```python
from build123d import *

# Parameters (mm, degrees)
SKETCH1_W           = 65
SKETCH1_H           = 57
SKETCH1_R           = 3.25
BOSS_EXTRUDE1_DEPTH = 21.5
CHAMFER1_SIZE       = 6
SKETCH2_W           = 13
SKETCH2_H           = 26
SKETCH2_H_2         = 5
CUT_EXTRUDE1_DEPTH  = 19.5
FILLET1_R           = 3


with BuildPart() as part:
    # Sketch1 → Boss-Extrude1 (new body)
    with BuildSketch(Plane(origin=(0, 0, 0), x_dir=(1, 0, 0), z_dir=(0, 1, 0))):
        Rectangle(SKETCH1_W, SKETCH1_H)
        with Locations((27.75, -2.25)):
            Circle(SKETCH1_R, mode=Mode.SUBTRACT)
        with Locations((-27.75, -2.25)):
            Circle(SKETCH1_R, mode=Mode.SUBTRACT)
    extrude(amount=BOSS_EXTRUDE1_DEPTH)

    # Chamfer1
    chamfer1_edges = [part.edges().sort_by_distance(p)[0] for p in [
        (32.5, 10.75, 28.5),
        (-32.5, 10.75, 28.5),
        (-32.5, 10.75, -28.5),
        (32.5, 10.75, -28.5),
    ]]
    chamfer(chamfer1_edges, length=CHAMFER1_SIZE)

    # Sketch2 → Cut-Extrude1 (cut)
    with BuildSketch(Plane(origin=(0, 21.5, 0), x_dir=(1, 0, 0), z_dir=(0, 1, 0))):
        with Locations((-26, 0)):
            Rectangle(SKETCH2_W, SKETCH2_H)
        with Locations((-26, 17.1)):
            Rectangle(SKETCH2_W, SKETCH2_H_2)
        with Locations((-26, 23.7)):
            Rectangle(SKETCH2_W, SKETCH2_H_2)
        with Locations((-26, -17.1)):
            Rectangle(SKETCH2_W, SKETCH2_H_2)
        with Locations((-26, -23.7)):
            Rectangle(SKETCH2_W, SKETCH2_H_2)
        with Locations((26, -23.7)):
            Rectangle(SKETCH2_W, SKETCH2_H_2)
        with Locations((26, -17.1)):
            Rectangle(SKETCH2_W, SKETCH2_H_2)
        with Locations((26, 0)):
            Rectangle(SKETCH2_W, SKETCH2_H)
        with Locations((26, 17.1)):
            Rectangle(SKETCH2_W, SKETCH2_H_2)
        with Locations((26, 23.7)):
            Rectangle(SKETCH2_W, SKETCH2_H_2)
    extrude(amount=-CUT_EXTRUDE1_DEPTH, mode=Mode.SUBTRACT)

    # Fillet1
    fillet1_edges = [part.edges().sort_by_distance(p)[0] for p in [
        (-19.5, 21.5, 17.1),
        (-19.5, 21.5, 23.7),
        (19.5, 21.5, 23.7),
        (19.5, 21.5, 17.1),
        (19.5, 21.5, 0),
        (19.5, 21.5, -17.1),
        (19.5, 21.5, -23.7),
        (-19.5, 21.5, 0),
        (-27.65, 21.5, -27.35),
        (27.65, 21.5, 27.35),
        (-27.65, 21.5, 27.35),
        (27.65, 21.5, -27.35),
        (-32.5, 21.5, -20.4),
        (-32.5, 21.5, -13.8),
        (-32.5, 21.5, 13.8),
        (-32.5, 21.5, 20.4),
        (32.5, 21.5, 20.4),
        (32.5, 21.5, 13.8),
        (32.5, 21.5, -13.8),
        (32.5, 21.5, -20.4),
        (-19.5, 21.5, -17.1),
        (-19.5, 21.5, -23.7),
    ]]
    fillet(fillet1_edges, radius=FILLET1_R)


solid = part.part
```
Could you check a few things on this model? Use its own coordinates, in mm. A direction names the side the tool comes from. Round coordinates to 2 decimals unless told otherwise and drop trailing zeros. Write each loop counter-clockwise with the first axis right and the second up, starting at its lowest first coordinate (ties: lowest second). Pieces come first, ordered by that corner, then holes. Notation, with made-up numbers: M 26,46 L 39,46 A27 cw 39,65 Z; hole C 82.5,60.25 d2. An arc over 180 degrees is marked long. Answer in a Markdown table with one row per item. Add a question column.
Q1. Will these pins go through, and if not, where does the flat tip stop? pin 1 Ø1.5 at (y, z) = (14, 16.5) entering from -X; pin 2 Ø4 at (x, z) = (-28, 1.5) entering from +Y; pin 3 Ø1.5 at (y, z) = (7.5, -16) entering from +X; pin 4 Ø2.5 at (x, z) = (24.5, -16.5) entering from +Y.
Q2. If I drill on line 1 (X direction, y = 1.1, z = 2.25); line 2 (Z direction, x = -22, y = 13.25); line 3 (X direction, y = 4.5, z = -4.5), over which ranges is the centre line in solid material (lowest first)? Write a range as from..to.
Q3. Imagine slicing it at A-A (z = 2.25). Please give me the cut outline in (x, y), then the cut area to 3 significant figures.
Q4. Imagine slicing it at B-B (z = -24). Please give me the cut outline in (x, y).
Q5. If we mould it in two halves opening along Z, with no side actions, what happens to faces 4 (the flat face through (32.5, 1.7, 0.1)), 5 (the flat face through (28, 7, 27)), 6 (the flat face through (19.5, 10, 24))? For each: +Z half, -Z half, draft (parallel to the pull), parting line (faces both ways), or undercut.
Q6. On a 3-axis mill with a long thin cutter (end or side, diameter ignored), from which of +Z, -Z, +X, -X, +Y, -Y can I reach the whole of each face in a straight line? I mean faces 1 (the cylindrical face through (18.6, 20.64, -0.18)), 2 (the flat face through (-26, 12, -19.6)), 3 (the flat face through (-28, 9, -27)). Say none if no direction works.
Values:
| question | item | result |
|---|---|---|
| 1 | pin 1 | x = -19.5 |
| 1 | pin 2 | through |
| 1 | pin 3 | x = 19.5 |
| 1 | pin 4 | y = 2 |
| 2 | line 1 | -32.5..-31, -24.5..24.5, 31..32.5 |
| 2 | line 2 | -28.5..-26.2, -21.2..-19.6, -14.6..-13, 13..14.6, 19.6..21.2, 26.2..28.5 |
| 2 | line 3 | -19.5..19.5 |
| 3 | outline | M -32.5,0 L -31,0 L -31,2 L -32.5,2 Z; M -24.5,0 L 24.5,0 L 24.5,2 L 19.5,2 L 19.5,18.5 A3 ccw 16.5,21.5 L -16.5,21.5 A3 ccw -19.5,18.5 L -19.5,2 L -24.5,2 Z; M 31,0 L 32.5,0 L 32.5,2 L 31,2 Z |
| 3 | area | 861 mm^2 |
| 4 | outline | M -31,0 L 31,0 L 31,2 L 19.5,2 L 19.5,18.5 A3 ccw 16.5,21.5 L -16.5,21.5 A3 ccw -19.5,18.5 L -19.5,2 L -31,2 Z |
| 5 | face 4 | draft |
| 5 | face 5 | +Z half |
| 5 | face 6 | undercut |
| 6 | face 1 | +X, +Y |
| 6 | face 2 | -X, +Y |
| 6 | face 3 | -Z, -X, +Y, -Y |
